from build123d import *

# Parameters (mm, degrees)
SKETCH_1_W          = 170
SKETCH_1_H          = 19.6
EXTRUDE_1_DEPTH     = 6.6
SKETCH_2_W          = 170
SKETCH_2_H          = 8.1
EXTRUDE_2_DEPTH     = 3.5
SKETCH_3_R          = 3
CUT_EXTRUDE_1_DEPTH = 87.157123907
CHAMFER_1_SIZE      = 4


with BuildPart() as part:
    # 草图1 → 凸台-拉伸1 (new body)
    with BuildSketch(Plane.XY):
        Rectangle(SKETCH_1_W, SKETCH_1_H)
    extrude(amount=EXTRUDE_1_DEPTH)

    # 草图2 → 凸台-拉伸2 (add)
    with BuildSketch(Plane.XY.offset(6.6)):
        Rectangle(SKETCH_2_W, SKETCH_2_H)
    extrude(amount=EXTRUDE_2_DEPTH)

    # 草图3 → 切除-拉伸1 (cut, through all)
    with BuildSketch(Plane.XY.offset(10.1)):
        with Locations((-72.247114829, 0)):
            Circle(SKETCH_3_R)
        with Locations((-17.653434016, 0)):
            Circle(SKETCH_3_R)
        with Locations(Location((17.653434016, 0, 0), (0, 0, 180))):
            Circle(SKETCH_3_R)
        with Locations(Location((72.247114829, 0, 0), (0, 0, 180))):
            Circle(SKETCH_3_R)
    extrude(amount=-CUT_EXTRUDE_1_DEPTH, mode=Mode.SUBTRACT)

    # 倒角1
    chamfer_1_edges = [part.edges().sort_by_distance(p)[0] for p in [
        (0, -9.8, 0),
        (0, 9.8, 0),
    ]]
    chamfer(chamfer_1_edges, length=CHAMFER_1_SIZE)


solid = part.part
The model under review builds one solid part; all positions refer to its coordinate system, in mm. A direction names the side the tool comes from. Give positions to 0.01 mm unless a question says otherwise; leave off trailing zeros. Order: outer loops, then holes, each group sorted by start corner. A loop starts at its lowest first (then second) coordinate and runs counter-clockwise, first axis right, second up. Notation, with made-up numbers: M -36.75,16.5 L -25.75,16.5 A30 ccw -25.75,51.5 Z; hole C 32,66 d1. An arc over 180 degrees is marked long. Use one line per item in the form item = value. Start each with the question number.
Item 1: We need section D-D on y = 8.25. Give the boundary of the cut face in (x, z), plus the area to 4 significant figures.
Item 2: To check wall thickness, follow line 1 along X through (y, z) = (-1.25, 3); line 2 along X through (y, z) = (-2.5, 7); line 3 along Z through (x, y) = (-2.5, 4.25). State the ranges of each line that lie inside material, in increasing order. Write a range as from..to.
Item 3: We need section A-A on y = 0. Give the boundary of the cut face in (x, z).
Item 4: For faces 1 (the flat face through (-1, -9.8, 5)), 2 (the flat face through (-1, 4.05, 8)), 3 (the flat face through (-1, -7, 6.6)), list the 3-axis set-ups (+Z, -Z, +X, -X, +Y, -Y) from which the entire face can be reached by the end or side of a thin tool; tool diameter is ignored.
Item 5: We need section B-B on z = 8.25. Give the boundary of the cut face in (x, y), plus the area to 3 significant figures.
Item 6: Insertion check: pin 1 Ø5.5 at (x, y) = (-17.65, 0) entering from -Z; pin 2 Ø1.5 at (x, z) = (5.5, 7.5) entering from -Y; pin 3 Ø4.5 at (x, y) = (-17.5, -6.5) entering from +Z. Each pin has a flat end and moves straight along its axis. Give the tip position at first contact, or say it passes through.
Item 7: We need section C-C on x = 36. Give the boundary of the cut face in (y, z).
Completed:
q1.outline = M -85,2.45 L 85,2.45 L 85,6.6 L -85,6.6 Z
q1.area = 705.5 mm²
q2.line_1 = -85..-74.97, -69.52..-20.38, -14.93..14.93, 20.38..69.52, 74.97..85
q2.line_2 = -85..-73.91, -70.59..-19.31, -16..16, 19.31..70.59, 73.91..85
q2.line_3 = 0..6.6
q3.outline = M -85,0 L -75.25,0 L -75.25,10.1 L -85,10.1 Z; M -69.25,0 L -20.65,0 L -20.65,10.1 L -69.25,10.1 Z; M -14.65,0 L 14.65,0 L 14.65,10.1 L -14.65,10.1 Z; M 20.65,0 L 69.25,0 L 69.25,10.1 L 20.65,10.1 Z; M 75.25,0 L 85,0 L 85,10.1 L 75.25,10.1 Z
q4.face_1 = +Z, -Z, +X, -X, -Y
q4.face_2 = +Z, +X, -X, +Y
q4.face_3 = +Z, +X, -X, -Y
q5.outline = M -85,-4.05 L 85,-4.05 L 85,4.05 L -85,4.05 Z; hole C -72.25,0 d6; hole C -17.65,0 d6; hole C 17.65,0 d6; hole C 72.25,0 d6
q5.area = 1,260 mm²
q6.pin_1 = through
q6.pin_2 = -4.05
q6.pin_3 = 6.6
q7.outline = M -9.8,4 L -5.8,0 L 5.8,0 L 9.8,4 L 9.8,6.6 L 4.05,6.6 L 4.05,10.1 L -4.05,10.1 L -4.05,6.6 L -9.8,6.6 Z
